```python
from build123d import *

# Parameters (mm, degrees)
BOSS_EXTRUDE1_DEPTH = 10
CUT_EXTRUDE1_DEPTH  = 50
SKETCH3_R           = 1.625
CUT_EXTRUDE2_DEPTH  = 6
SKETCH8_R           = 2.45
CUT_EXTRUDE3_DEPTH  = 6


with BuildPart() as part:
    # Sketch1 → Boss-Extrude1 (new body, symmetric)
    with BuildSketch(Plane.XY):
        with BuildLine():
            Line((0, 0), (0, 130))
            Line((0, 130), (-2, 130))
            ThreePointArc((-2, 130), (-4.121320344, 129.121320344), (-5, 127))
            Line((-5, 127), (-5, 11))
            ThreePointArc((-5, 11), (-6.757359313, 6.757359313), (-11, 5))
            Line((-11, 5), (-47, 5))
            ThreePointArc((-47, 5), (-49.121320344, 4.121320344), (-50, 2))
            Line((-50, 2), (-50, 0))
            Line((-50, 0), (0, 0))
        make_face()
    extrude(amount=BOSS_EXTRUDE1_DEPTH, both=True)

    # Sketch2 → Cut-Extrude1 (cut)
    with BuildSketch(Plane(origin=(0, 130, 0), x_dir=(1, 0, 0), z_dir=(0, 1, 0))):
        with BuildLine():
            ThreePointArc((0, 10), (-0.884048614, 0), (0, -10))
            Line((0, -10), (0, 10))
        make_face()
        with BuildLine():
            Line((0, 10), (0, -10))
            ThreePointArc((0, -10), (61.135451908, -56.7785577), (113.115951386, 0))
            ThreePointArc((113.115951386, 0), (61.135451908, 56.7785577), (0, 10))
        make_face()
    extrude(amount=-CUT_EXTRUDE1_DEPTH, mode=Mode.SUBTRACT)

    # Sketch3 → Cut-Extrude2 (cut, through all)
    with BuildSketch(Plane.ZY.offset(5)):
        with Locations((0, 93.5)):
            Circle(SKETCH3_R)
        with Locations((0, 113.5)):
            Circle(SKETCH3_R)
    extrude(amount=-CUT_EXTRUDE2_DEPTH, mode=Mode.SUBTRACT)

    # Sketch8 → Cut-Extrude3 (cut, through all)
    with BuildSketch(Plane(origin=(0, 5, 0), x_dir=(1, 0, 0), z_dir=(0, 1, 0))):
        with Locations((-29, 0)):
            Circle(SKETCH8_R)
    extrude(amount=-CUT_EXTRUDE3_DEPTH, mode=Mode.SUBTRACT)


solid = part.part
```
Verification items for the finished model (mm, model axes). A direction names the side the tool comes from. Coordinates: 2 decimals unless noted, no trailing zeros. Loops run counter-clockwise (first coordinate to the right, second up) from the corner with the lowest first, then second, coordinate; pieces in that order, holes last. Notation, with made-up numbers: (46, -7.75) -> (75, -7.75) arc R20 cw to (75, 6.25) -> close; hole circle Ø1 at (67.5, 5). An arc over 180 degrees is marked (long way). Answer in a Markdown table with one row per item.
1) Draft check along Z on faces 4 (the face through (-6.711, 6.804, 0.14)), 5 (the face through (-26.663, 2.535, -0.736)), 6 (the face through (-4.7, 46, 10)). Enter one of: released by +Z, released by -Z, zero draft, split by the parting line, or undercut.
The answers:
| item | result |
|---|---|
| face 4 | zero draft |
| face 5 | undercut |
| face 6 | released by +Z |
2) Section check A-A (y = 93.5). Record the cut outline in (x, z) (3 decimals).
The answers:
| item | result |
|---|---|
| outline | (-5, -10) -> (0, -10) arc R57 cw to (-0.861, -1.625) -> (-5, -1.625) -> close; (-5, 1.625) -> (-0.861, 1.625) arc R57 cw to (0, 10) -> (-5, 10) -> close |
3) Section check D-D (z = 6.25). Record the cut outline in (x, y).
The answers:
| item | result |
|---|---|
| outline | (-50, 0) -> (0, 0) -> (0, 80) -> (-0.54, 80) -> (-0.54, 130) -> (-2, 130) arc R3 ccw to (-5, 127) -> (-5, 11) arc R6 cw to (-11, 5) -> (-47, 5) arc R3 ccw to (-50, 2) -> close |
4) Depth check by flat-ended pin: P1, Ø5, axis at y = 113.5, z = 0, coming from the +X side; P2, Ø6, axis at x = -21.5, z = -2.5, coming from the +Y side; P3, Ø1, axis at y = 76, z = -3, coming from the -X side. Enter the tip coordinate at first touch or a pass-through.
The answers:
| item | result |
|---|---|
| P1 | stops at x = -0.83 |
| P2 | stops at y = 5 |
| P3 | stops at x = -5 |
5) Access from +Z, -Z, +X, -X, +Y, -Y to the whole of each face (thin tool, end or side, straight path). Record for faces 1 (the face through (-4.7, 46, -10)), 2 (the face through (-5, 70, 0)), 3 (the face through (-0.884, 105.35, -0.141)).
The answers:
| item | result |
|---|---|
| face 1 | -Z, +X, -X, +Y, -Y |
| face 2 | +Z, -Z, -X, +Y |
| face 3 | +X, +Y |
6) Scan lines: line 1 along Z through (x, y) = (-29, 2.1); line 2 along Z through (x, y) = (-4, 93.5) (3 decimals); line 3 along Y through (x, z) = (-3.3, 0) (3 decimals). Record each from-to range of solid material in increasing order. Write a range as from..to.
The answers:
| item | result |
|---|---|
| line 1 | z = -10..-2.45, 2.45..10 |
| line 2 | z = -10..-1.625, 1.625..10 |
| line 3 | y = 0..91.875, 95.125..111.875, 115.125..129.704 |
7) Section check B-B (z = 0). Record the cut outline in (x, y) (3 decimals).
The answers:
| item | result |
|---|---|
| outline | (-50, 0) -> (-31.45, 0) -> (-31.45, 5) -> (-47, 5) arc R3 ccw to (-50, 2) -> close; (-26.55, 0) -> (0, 0) -> (0, 80) -> (-0.884, 80) -> (-0.884, 91.875) -> (-5, 91.875) -> (-5, 11) arc R6 cw to (-11, 5) -> (-26.55, 5) -> close; (-5, 95.125) -> (-0.884, 95.125) -> (-0.884, 111.875) -> (-5, 111.875) -> close; (-5, 115.125) -> (-0.884, 115.125) -> (-0.884, 130) -> (-2, 130) arc R3 ccw to (-5, 127) -> close |
8) Section check C-C (x = -29). Record the cut outline in (y, z).
The answers:
| item | result |
|---|---|
| outline | (0, -10) -> (5, -10) -> (5, -2.45) -> (0, -2.45) -> close; (0, 2.45) -> (5, 2.45) -> (5, 10) -> (0, 10) -> close |
